```python
from build123d import *

# Parameters (mm, degrees)
SKETCH1_W           = 10.922
SKETCH1_H           = 18.542
BOSS_EXTRUDE1_DEPTH = 1.524
SKETCH3_R           = 5.461
SKETCH3_R_2         = 1.778
BOSS_EXTRUDE2_DEPTH = 8.89
SKETCH2_W           = 13.462
SKETCH2_H           = 21.082
SKETCH2_W_2         = 10.922
SKETCH2_H_2         = 18.542
EXTRUDE_THIN1_DEPTH = 7.62
CUT_EXTRUDE1_START  = -20.32
SKETCH4_R           = 1.778
CUT_EXTRUDE1_DEPTH  = 20.32
FILLET1_R           = 1.27
FILLET2_R           = 0.762
FILLET3_R           = 0.762
CUT_EXTRUDE2_DEPTH  = 0.635


with BuildPart() as part:
    # Sketch1 → Boss-Extrude1 (new body)
    with BuildSketch(Plane.XY):
        Rectangle(SKETCH1_W, SKETCH1_H)
    extrude(amount=BOSS_EXTRUDE1_DEPTH)

    # Sketch3 → Boss-Extrude2 (add)
    with BuildSketch(Plane.XY):
        with Locations((0, 0.508)):
            Circle(SKETCH3_R)
        with Locations((0, 0.508)):
            Circle(SKETCH3_R_2, mode=Mode.SUBTRACT)
    extrude(amount=-BOSS_EXTRUDE2_DEPTH)

    # Sketch2 → Extrude-Thin1 (add)
    with BuildSketch(Plane.XY):
        Rectangle(SKETCH2_W, SKETCH2_H)
        Rectangle(SKETCH2_W_2, SKETCH2_H_2, mode=Mode.SUBTRACT)
    extrude(amount=EXTRUDE_THIN1_DEPTH)

    # Sketch4 → Cut-Extrude1 (cut)
    with BuildSketch(Plane(origin=(0, 0, -8.89), x_dir=(-1, 0, 0), z_dir=(0, 0, -1)).offset(CUT_EXTRUDE1_START)):
        with Locations(Location((0, 0.508, 0), (0, 0, 180))):
            Circle(SKETCH4_R)
    extrude(amount=CUT_EXTRUDE1_DEPTH, mode=Mode.SUBTRACT)

    # Fillet1
    fillet1_edges = [part.edges().sort_by_distance(p)[0] for p in [
        (-5.461, 0.508, 0),
        (6.731, -10.541, 3.81),
        (6.731, 10.541, 3.81),
        (-6.731, 10.541, 3.81),
    ]]
    fillet(fillet1_edges, radius=FILLET1_R - 0.0001)  # a hair under: the kernel refuses the full size

    # Fillet2
    fillet2_edges = [part.edges().sort_by_distance(p)[0] for p in [
        (-5.461, 0.508, -8.89),
    ]]
    fillet(fillet2_edges, radius=FILLET2_R)

    # Fillet3
    fillet3_edges = [part.edges().sort_by_distance(p)[0] for p in [
        (-0.63495, -10.541, 0),
        (6.731, 0, 0),
        (6.731, 0, 0),
        (-6.731, -0.63495, 0),
        (-6.731, -0.63495, 0),
        (0, 10.541, 0),
        (-6.359054901, 10.169054901, 0),
        (6.359054901, 10.169054901, 0),
        (6.359054901, -10.169054901, 0),
    ]]
    fillet(fillet3_edges, radius=FILLET3_R)

    # Sketch5 → Cut-Extrude2 (cut)
    with BuildSketch(Plane(origin=(0, 0, 0), x_dir=(-1, 0, 0), z_dir=(0, 0, -1))):
        Polygon((3.390564192, -7.848738261), (5.164036584, -8.872653024), (5.164036584, -6.824823498), align=None)
    extrude(amount=-CUT_EXTRUDE2_DEPTH, mode=Mode.SUBTRACT)


solid = part.part
```
Check sheet for the modelled part. Datum: model origin and axes. Units: mm. A direction names the side the tool comes from. Give positions to 0.01 mm unless a question says otherwise; leave off trailing zeros. Write each loop counter-clockwise with the first axis right and the second up, starting at its lowest first coordinate (ties: lowest second). Pieces come first, ordered by that corner, then holes.
Item 1: Access from +Z, -Z, +X, -X, +Y, -Y to the whole of each face (thin tool, end or side, straight path). Record for faces 4 (the face through (0, 8, 0)), 5 (the face through (0, -2, 1.524)), 6 (the face through (6.37, 10.16, 4.24)), 7 (the face through (-4.26, -8.35, 0.31)), 8 (the face through (-6, 0, 7.62)).
Item 2: Gauge pin test, flat ends, axial feed: pin 1 (1.4 mm diameter, centred on x = -4.5, y = -7.5, fed in from -Z); pin 2 (2 mm diameter, centred on x = -1, y = -7, fed in from +Z). Record the tip position at first contact, or that the pin passes through.
Item 3: Draft check along Y on faces 1 (the face through (0, -9.271, 5)), 2 (the face through (-1, -10.541, 4)), 3 (the face through (-6.37, 10.16, 4.24)). Enter one of: released by +Y, released by -Y, zero draft, split by the parting line, or undercut.
Item 4: Scan lines: L1, parallel to X at y = -8, z = 4; L2, parallel to Y at x = -1.5, z = 2.5; L3, parallel to Z at x = -3.25, y = -0.75. Record each from-to range of solid material in increasing order.
Item 5: Cross-section at A-A (x = 0). Enter the section's corners in (y, z), and give its area (3 significant figures).
Item 6: Cross-section at C-C (z = -2). Enter the section's corners in (x, y).
Item 7: Cross-section at B-B (z = 2). Enter the section's corners in (x, y), and give its area (3 significant figures).
Report:
1. face 4: -Z, +Y
1. face 5: +Z
1. face 6: +Z, -Z, +X, +Y
1. face 7: -Z
1. face 8: +Z, +X, -X, +Y, -Y
2. pin 1: stops at z = 0
2. pin 2: stops at z = 1.52
3. face 1: undercut
3. face 2: released by -Y
3. face 3: released by +Y
4. L1: x = -6.73 to -5.46, 5.46 to 6.73
4. L2: y = -10.54 to -9.27, 9.27 to 10.54
4. L3: z = -8.89 to 1.52
5. outline: (-10.54, 0.76) arc R0.76 ccw to (-9.78, 0) - (-6.22, 0) arc R1.27 cw to (-4.95, -1.27) - (-4.95, -8.13) arc R0.76 ccw to (-4.19, -8.89) - (-1.27, -8.89) - (-1.27, 1.52) - (-9.27, 1.52) - (-9.27, 7.62) - (-10.54, 7.62) - close; (2.29, -8.89) - (5.21, -8.89) arc R0.76 ccw to (5.97, -8.13) - (5.97, -1.27) arc R1.27 cw to (7.24, 0) - (9.78, 0) arc R0.76 ccw to (10.54, 0.76) - (10.54, 7.62) - (9.27, 7.62) - (9.27, 1.52) - (2.29, 1.52) - close
5. area: 108 mm2
6. outline: circle Ø10.92 at (0, 0.51); hole circle Ø3.56 at (0, 0.51)
7. outline: (-6.73, -10.54) - (5.46, -10.54) arc R1.27 ccw to (6.73, -9.27) - (6.73, 9.27) arc R1.27 ccw to (5.46, 10.54) - (-5.46, 10.54) arc R1.27 ccw to (-6.73, 9.27) - close; hole (-5.46, -9.27) - (5.46, -9.27) - (5.46, 9.27) - (-5.46, 9.27) - close
7. area: 80.3 mm2
